Drawing for the job (mm, zero at the part's lowest x, y, z). A direction names the side the tool comes from. Give positions to 0.01 mm unless a question says otherwise; leave off trailing zeros. Write each loop counter-clockwise with the first axis right and the second up, starting at its lowest first coordinate (ties: lowest second). Pieces come first, ordered by that corner, then holes.
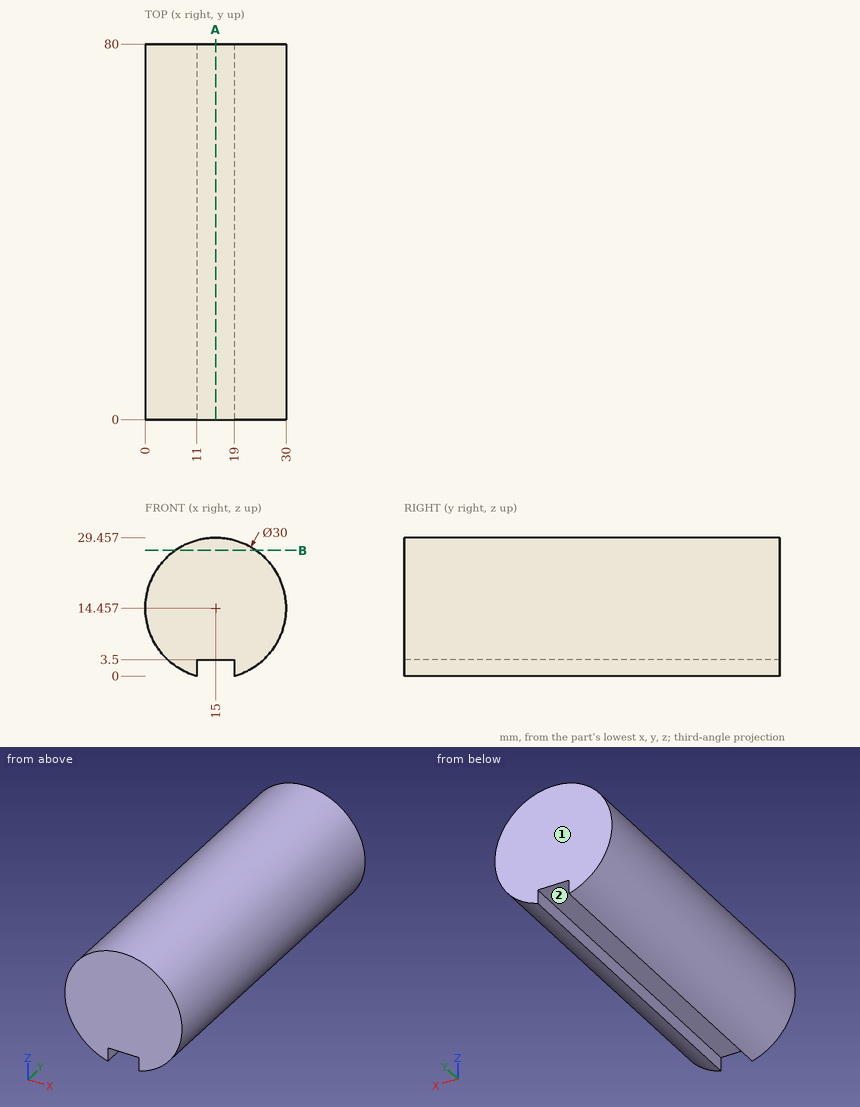
1. Which spindle directions (+Z, -Z, +X, -X, +Y, -Y) get a long thin tool onto all of the face, cutting with end or side? Do the marked faces 1 and 2. Say none if no direction does.
Calculated:
face 1: +Z, -Z, +X, -X, +Y
face 2: -Z, +Y, -Y
2. Slice it at B-B, the plane z = 26.75. Write the cut outline in (x, y) (1 decimal), and give its area (3 significant figures).
Calculated:
outline: (6.4, 0) - (23.6, 0) - (23.6, 80) - (6.4, 80) - close
area: 1,380 mm2
3. Probe probe 1 along Z at (x, y) = (14.5, 32); probe 2 along X at (y, z) = (29, 2) (1 decimal); probe 3 along X at (y, z) = (16, 12.75). List the from-to ranges inside material, lowest first.
Calculated:
probe 1: z = 3.5 to 29.45
probe 2: x = 6.6 to 11, 19 to 23.4
probe 3: x = 0.1 to 29.9
4. Slice it at A-A, the plane x = 15. Write the cut outline in (y, z).
Calculated:
outline: (0, 3.5) - (80, 3.5) - (80, 29.46) - (0, 29.46) - close
5. Pin check, flat tips, straight feed: P1, Ø1, axis at y = 57, z = 2, coming from the +X side; P2, Ø2, axis at x = 9, y = 58, coming from the +Z side; P3, Ø3, axis at y = 20.5, z = 1, coming from the -X side; P4, Ø1, axis at x = 27, z = 24.5, coming from the +Y side. Stop position of each tip, or through.
Calculated:
P1: stops at x = 24.06
P2: stops at z = 28.6
P3: stops at x = 5.94
P4: passes through
